The model under review builds one solid part; all positions refer to its coordinate system, in mm. Coordinates: 2 decimals unless noted, no trailing zeros. Loops run counter-clockwise (first coordinate to the right, second up) from the corner with the lowest first, then second, coordinate; pieces in that order, holes last. Notation, with made-up numbers: M -13.5,70.5 L -6.5,70.5 A29 ccw -6.5,92.5 Z; hole C -2.5,49.25 d6. An arc over 180 degrees is marked long. Return JSON: item names as keys, results as strings.
```python
from build123d import *

# Parameters (mm, degrees)
SKETCH1_R           = 2.0701
BOSS_EXTRUDE1_DEPTH = 3.175


with BuildPart() as part:
    # Sketch1 → Boss-Extrude1 (new body)
    with BuildSketch(Plane.XY):
        Polygon((317.5, 546.1), (190.5, 546.1), (88.9, 647.7), (88.9, 774.7), (-215.9, 774.7), (-215.9, 647.7), (-317.5, 546.1), (-444.5, 546.1), (-444.5, 241.3), (-317.5, 241.3), (-215.9, 139.7), (-215.9, 12.7), (88.9, 12.7), (88.9, 139.7), (190.5, 241.3), (317.5, 241.3), align=None)
        with Locations((76.2, 762)):
            Circle(SKETCH1_R, mode=Mode.SUBTRACT)
        with Locations((50.8, 762)):
            Circle(SKETCH1_R, mode=Mode.SUBTRACT)
        with Locations((25.4, 762)):
            Circle(SKETCH1_R, mode=Mode.SUBTRACT)
        with Locations((0, 762)):
            Circle(SKETCH1_R, mode=Mode.SUBTRACT)
        with Locations((-25.4, 762)):
            Circle(SKETCH1_R, mode=Mode.SUBTRACT)
        with Locations((-50.8, 762)):
            Circle(SKETCH1_R, mode=Mode.SUBTRACT)
        with Locations((-76.2, 762)):
            Circle(SKETCH1_R, mode=Mode.SUBTRACT)
        with Locations((-101.6, 762)):
            Circle(SKETCH1_R, mode=Mode.SUBTRACT)
        with Locations((-127, 762)):
            Circle(SKETCH1_R, mode=Mode.SUBTRACT)
        with Locations((-152.4, 762)):
            Circle(SKETCH1_R, mode=Mode.SUBTRACT)
        with Locations((-177.8, 762)):
            Circle(SKETCH1_R, mode=Mode.SUBTRACT)
        with Locations((-203.2, 762)):
            Circle(SKETCH1_R, mode=Mode.SUBTRACT)
        with Locations(Location((76.2, 25.4, 0), (0, 0, 180))):
            Circle(SKETCH1_R, mode=Mode.SUBTRACT)
        with Locations(Location((50.8, 25.4, 0), (0, 0, 180))):
            Circle(SKETCH1_R, mode=Mode.SUBTRACT)
        with Locations(Location((-50.8, 25.4, 0), (0, 0, 180))):
            Circle(SKETCH1_R, mode=Mode.SUBTRACT)
        with Locations(Location((-25.4, 25.4, 0), (0, 0, 180))):
            Circle(SKETCH1_R, mode=Mode.SUBTRACT)
        with Locations(Location((0, 25.4, 0), (0, 0, 180))):
            Circle(SKETCH1_R, mode=Mode.SUBTRACT)
        with Locations(Location((25.4, 25.4, 0), (0, 0, 180))):
            Circle(SKETCH1_R, mode=Mode.SUBTRACT)
        with Locations(Location((-76.2, 25.4, 0), (0, 0, 180))):
            Circle(SKETCH1_R, mode=Mode.SUBTRACT)
        with Locations(Location((-101.6, 25.4, 0), (0, 0, 180))):
            Circle(SKETCH1_R, mode=Mode.SUBTRACT)
        with Locations(Location((-127, 25.4, 0), (0, 0, 180))):
            Circle(SKETCH1_R, mode=Mode.SUBTRACT)
        with Locations(Location((-152.4, 25.4, 0), (0, 0, 180))):
            Circle(SKETCH1_R, mode=Mode.SUBTRACT)
        with Locations(Location((-177.8, 25.4, 0), (0, 0, 180))):
            Circle(SKETCH1_R, mode=Mode.SUBTRACT)
        with Locations(Location((-203.2, 25.4, 0), (0, 0, 180))):
            Circle(SKETCH1_R, mode=Mode.SUBTRACT)
        with Locations(Location((-152.4, 50.8, 0), (0, 0, 180))):
            Circle(SKETCH1_R, mode=Mode.SUBTRACT)
        with Locations(Location((-152.4, 76.2, 0), (0, 0, 180))):
            Circle(SKETCH1_R, mode=Mode.SUBTRACT)
        with Locations(Location((-152.4, 101.6, 0), (0, 0, 180))):
            Circle(SKETCH1_R, mode=Mode.SUBTRACT)
        with Locations(Location((-152.4, 127, 0), (0, 0, 180))):
            Circle(SKETCH1_R, mode=Mode.SUBTRACT)
        with Locations(Location((-152.4, 152.4, 0), (0, 0, 180))):
            Circle(SKETCH1_R, mode=Mode.SUBTRACT)
        with Locations(Location((-152.4, 177.8, 0), (0, 0, 180))):
            Circle(SKETCH1_R, mode=Mode.SUBTRACT)
        with Locations(Location((-152.4, 203.2, 0), (0, 0, 180))):
            Circle(SKETCH1_R, mode=Mode.SUBTRACT)
        with Locations(Location((-152.4, 228.6, 0), (0, 0, 180))):
            Circle(SKETCH1_R, mode=Mode.SUBTRACT)
        with Locations(Location((-152.4, 254, 0), (0, 0, 180))):
            Circle(SKETCH1_R, mode=Mode.SUBTRACT)
        with Locations(Location((-152.4, 279.4, 0), (0, 0, 180))):
            Circle(SKETCH1_R, mode=Mode.SUBTRACT)
        with Locations(Location((-152.4, 304.8, 0), (0, 0, 180))):
            Circle(SKETCH1_R, mode=Mode.SUBTRACT)
        with Locations(Location((-152.4, 330.2, 0), (0, 0, 180))):
            Circle(SKETCH1_R, mode=Mode.SUBTRACT)
        with Locations(Location((-152.4, 355.6, 0), (0, 0, 180))):
            Circle(SKETCH1_R, mode=Mode.SUBTRACT)
        with Locations(Location((-152.4, 381, 0), (0, 0, 180))):
            Circle(SKETCH1_R, mode=Mode.SUBTRACT)
        with Locations(Location((-152.4, 406.4, 0), (0, 0, 180))):
            Circle(SKETCH1_R, mode=Mode.SUBTRACT)
        with Locations(Location((-152.4, 431.8, 0), (0, 0, 180))):
            Circle(SKETCH1_R, mode=Mode.SUBTRACT)
        with Locations(Location((-152.4, 457.2, 0), (0, 0, 180))):
            Circle(SKETCH1_R, mode=Mode.SUBTRACT)
        with Locations(Location((-152.4, 482.6, 0), (0, 0, 180))):
            Circle(SKETCH1_R, mode=Mode.SUBTRACT)
        with Locations(Location((-152.4, 508, 0), (0, 0, 180))):
            Circle(SKETCH1_R, mode=Mode.SUBTRACT)
        with Locations(Location((-152.4, 533.4, 0), (0, 0, 180))):
            Circle(SKETCH1_R, mode=Mode.SUBTRACT)
        with Locations(Location((-152.4, 558.8, 0), (0, 0, 180))):
            Circle(SKETCH1_R, mode=Mode.SUBTRACT)
        with Locations(Location((-152.4, 584.2, 0), (0, 0, 180))):
            Circle(SKETCH1_R, mode=Mode.SUBTRACT)
        with Locations(Location((-152.4, 609.6, 0), (0, 0, 180))):
            Circle(SKETCH1_R, mode=Mode.SUBTRACT)
        with Locations(Location((-152.4, 635, 0), (0, 0, 180))):
            Circle(SKETCH1_R, mode=Mode.SUBTRACT)
        with Locations(Location((-152.4, 660.4, 0), (0, 0, 180))):
            Circle(SKETCH1_R, mode=Mode.SUBTRACT)
        with Locations(Location((-152.4, 685.8, 0), (0, 0, 180))):
            Circle(SKETCH1_R, mode=Mode.SUBTRACT)
        with Locations(Location((-152.4, 711.2, 0), (0, 0, 180))):
            Circle(SKETCH1_R, mode=Mode.SUBTRACT)
        with Locations(Location((-152.4, 736.6, 0), (0, 0, 180))):
            Circle(SKETCH1_R, mode=Mode.SUBTRACT)
        with Locations(Location((0, 50.8, 0), (0, 0, 180))):
            Circle(SKETCH1_R, mode=Mode.SUBTRACT)
        with Locations(Location((0, 76.2, 0), (0, 0, 180))):
            Circle(SKETCH1_R, mode=Mode.SUBTRACT)
        with Locations(Location((0, 101.6, 0), (0, 0, 180))):
            Circle(SKETCH1_R, mode=Mode.SUBTRACT)
        with Locations(Location((0, 127, 0), (0, 0, 180))):
            Circle(SKETCH1_R, mode=Mode.SUBTRACT)
        with Locations(Location((0, 152.4, 0), (0, 0, 180))):
            Circle(SKETCH1_R, mode=Mode.SUBTRACT)
        with Locations(Location((0, 177.8, 0), (0, 0, 180))):
            Circle(SKETCH1_R, mode=Mode.SUBTRACT)
        with Locations(Location((0, 203.2, 0), (0, 0, 180))):
            Circle(SKETCH1_R, mode=Mode.SUBTRACT)
        with Locations(Location((0, 228.6, 0), (0, 0, 180))):
            Circle(SKETCH1_R, mode=Mode.SUBTRACT)
        with Locations(Location((0, 254, 0), (0, 0, 180))):
            Circle(SKETCH1_R, mode=Mode.SUBTRACT)
        with Locations(Location((0, 279.4, 0), (0, 0, 180))):
            Circle(SKETCH1_R, mode=Mode.SUBTRACT)
        with Locations(Location((0, 304.8, 0), (0, 0, 180))):
            Circle(SKETCH1_R, mode=Mode.SUBTRACT)
        with Locations(Location((0, 330.2, 0), (0, 0, 180))):
            Circle(SKETCH1_R, mode=Mode.SUBTRACT)
        with Locations(Location((0, 355.6, 0), (0, 0, 180))):
            Circle(SKETCH1_R, mode=Mode.SUBTRACT)
        with Locations(Location((0, 381, 0), (0, 0, 180))):
            Circle(SKETCH1_R, mode=Mode.SUBTRACT)
        with Locations(Location((0, 406.4, 0), (0, 0, 180))):
            Circle(SKETCH1_R, mode=Mode.SUBTRACT)
        with Locations(Location((0, 431.8, 0), (0, 0, 180))):
            Circle(SKETCH1_R, mode=Mode.SUBTRACT)
        with Locations(Location((0, 457.2, 0), (0, 0, 180))):
            Circle(SKETCH1_R, mode=Mode.SUBTRACT)
        with Locations(Location((0, 482.6, 0), (0, 0, 180))):
            Circle(SKETCH1_R, mode=Mode.SUBTRACT)
        with Locations(Location((0, 508, 0), (0, 0, 180))):
            Circle(SKETCH1_R, mode=Mode.SUBTRACT)
        with Locations(Location((0, 533.4, 0), (0, 0, 180))):
            Circle(SKETCH1_R, mode=Mode.SUBTRACT)
        with Locations(Location((0, 558.8, 0), (0, 0, 180))):
            Circle(SKETCH1_R, mode=Mode.SUBTRACT)
        with Locations(Location((0, 584.2, 0), (0, 0, 180))):
            Circle(SKETCH1_R, mode=Mode.SUBTRACT)
        with Locations(Location((0, 609.6, 0), (0, 0, 180))):
            Circle(SKETCH1_R, mode=Mode.SUBTRACT)
        with Locations(Location((0, 635, 0), (0, 0, 180))):
            Circle(SKETCH1_R, mode=Mode.SUBTRACT)
        with Locations(Location((0, 660.4, 0), (0, 0, 180))):
            Circle(SKETCH1_R, mode=Mode.SUBTRACT)
        with Locations(Location((0, 685.8, 0), (0, 0, 180))):
            Circle(SKETCH1_R, mode=Mode.SUBTRACT)
        with Locations(Location((0, 711.2, 0), (0, 0, 180))):
            Circle(SKETCH1_R, mode=Mode.SUBTRACT)
        with Locations(Location((0, 736.6, 0), (0, 0, 180))):
            Circle(SKETCH1_R, mode=Mode.SUBTRACT)
        with Locations((-431.8, 533.4)):
            Circle(SKETCH1_R, mode=Mode.SUBTRACT)
        with Locations((-431.8, 508)):
            Circle(SKETCH1_R, mode=Mode.SUBTRACT)
        with Locations((-431.8, 482.6)):
            Circle(SKETCH1_R, mode=Mode.SUBTRACT)
        with Locations((-431.8, 457.2)):
            Circle(SKETCH1_R, mode=Mode.SUBTRACT)
        with Locations((-431.8, 431.8)):
            Circle(SKETCH1_R, mode=Mode.SUBTRACT)
        with Locations((-431.8, 406.4)):
            Circle(SKETCH1_R, mode=Mode.SUBTRACT)
        with Locations((-431.8, 381)):
            Circle(SKETCH1_R, mode=Mode.SUBTRACT)
        with Locations((-431.8, 355.6)):
            Circle(SKETCH1_R, mode=Mode.SUBTRACT)
        with Locations((-431.8, 330.2)):
            Circle(SKETCH1_R, mode=Mode.SUBTRACT)
        with Locations((-431.8, 304.8)):
            Circle(SKETCH1_R, mode=Mode.SUBTRACT)
        with Locations((-431.8, 279.4)):
            Circle(SKETCH1_R, mode=Mode.SUBTRACT)
        with Locations((-431.8, 254)):
            Circle(SKETCH1_R, mode=Mode.SUBTRACT)
        with Locations(Location((304.8, 254, 0), (0, 0, 180))):
            Circle(SKETCH1_R, mode=Mode.SUBTRACT)
        with Locations(Location((304.8, 279.4, 0), (0, 0, 180))):
            Circle(SKETCH1_R, mode=Mode.SUBTRACT)
        with Locations(Location((304.8, 304.8, 0), (0, 0, 180))):
            Circle(SKETCH1_R, mode=Mode.SUBTRACT)
        with Locations(Location((304.8, 330.2, 0), (0, 0, 180))):
            Circle(SKETCH1_R, mode=Mode.SUBTRACT)
        with Locations(Location((304.8, 355.6, 0), (0, 0, 180))):
            Circle(SKETCH1_R, mode=Mode.SUBTRACT)
        with Locations(Location((304.8, 381, 0), (0, 0, 180))):
            Circle(SKETCH1_R, mode=Mode.SUBTRACT)
        with Locations(Location((304.8, 406.4, 0), (0, 0, 180))):
            Circle(SKETCH1_R, mode=Mode.SUBTRACT)
        with Locations(Location((304.8, 431.8, 0), (0, 0, 180))):
            Circle(SKETCH1_R, mode=Mode.SUBTRACT)
        with Locations(Location((304.8, 457.2, 0), (0, 0, 180))):
            Circle(SKETCH1_R, mode=Mode.SUBTRACT)
        with Locations(Location((304.8, 482.6, 0), (0, 0, 180))):
            Circle(SKETCH1_R, mode=Mode.SUBTRACT)
        with Locations(Location((304.8, 508, 0), (0, 0, 180))):
            Circle(SKETCH1_R, mode=Mode.SUBTRACT)
        with Locations(Location((304.8, 533.4, 0), (0, 0, 180))):
            Circle(SKETCH1_R, mode=Mode.SUBTRACT)
    extrude(amount=BOSS_EXTRUDE1_DEPTH)


solid = part.part
```
1. Add section C-C on x = -341.5. Give the boundary of the cut face in (y, z) (3 decimals).
Check values:
{"outline": "M 241.3,0 L 546.1,0 L 546.1,3.175 L 241.3,3.175 Z"}
2. To check wall thickness, follow line 1 (X direction, y = 660.4, z = 1.85); line 2 (X direction, y = 279.4, z = 1.2); line 3 (X direction, y = 280, z = 0.4). State the ranges of each line that lie inside material, in increasing order.
Check values:
{"line 1": "-215.9 to -154.47, -150.33 to -2.07, 2.07 to 88.9", "line 2": "-444.5 to -433.87, -429.73 to -154.47, -150.33 to -2.07, 2.07 to 302.73, 306.87 to 317.5", "line 3": "-444.5 to -433.78, -429.82 to -154.38, -150.42 to -1.98, 1.98 to 302.82, 306.78 to 317.5"}
3. Add section B-B on x = 149. Give the boundary of the cut face in (y, z) (3 decimals), plus the area to 3 significant figures.
Check values:
{"outline": "M 199.8,0 L 587.6,0 L 587.6,3.175 L 199.8,3.175 Z", "area": "1,230 mm²"}
4. Add section A-A on z = 0.95. State how many separate pieces and enclosed holes the cut face has, plus the area to 3 significant figures.
Check values:
{"separate pieces": "1", "enclosed holes": "104", "area": "391,000 mm²"}
